Autodesk Inventor part; units mm, degrees
ref_plane "YZ Plane" through (0, 0, 0) normal (1, 0, 0) x (0, 1, 0)
ref_plane "XZ Plane" through (0, 0, 0) normal (0, 1, 0) x (-1, 0, 0)
ref_plane "XY Plane" through (0, 0, 0) normal (0, 0, 1) x (1, 0, 0)
sketch "Boceto1" plane through (0, 0, 0) normal (0, 1, 0) x (-1, 0, 0)
  circle A0 centre (0, 0) radius 5
  circle A1 centre (0, 0) radius 1.5
  dimension "d0" = 10
  dimension "d1" = 3
extrude "Extrusión1" add sketch "Boceto1" along normal blind 10
sketch "Boceto2" plane through (0, 10, 0) normal (0, 1, 0) x (1, 0, 0)
  circle A0 centre (0, 0) radius 11
  circle A1 centre (0, 0) radius 5
  circle A2 centre (0, 0) radius 1.5
  dimension "d4" = 22
extrude "Extrusión2" add sketch "Boceto2" along normal blind 2.2 contours A0 | A1
sketch "Boceto3" plane through (0, 12.2, 0) normal (0, 1, 0) x (1, 0, 0)
  circle A0 centre (0, 0) radius 9.475
  circle A1 centre (0, 0) radius 6.6
  line L0 (0, -6.6) -> (0, -9.475)
  circle A2 centre (0, -8.0375) radius 1.4375
  circle A3 centre (8.0375, 0) radius 1.4375
  circle A4 centre (0, 8.0375) radius 1.4375
  circle A5 centre (-8.0375, 0) radius 1.4375
  dimension "d7" = 18.95
  dimension "d8" = 13.2
  dimension "d11" = 360
hole "Agujero1" at (0, 12.2, 8.0375) at (-8.0375, 12.2, 0) at (0, 12.2, -8.0375) at (8.0375, 12.2, 0) direction (0, -1, 0) diameter 2.85 end through all
properties part number "Acople motor" material "Hierro, dúctil"
The listing builds one solid part. Answer for the finished solid, in the listing's coordinates (mm). A direction names the side the tool comes from. Coordinates: 2 decimals unless noted, no trailing zeros. Loops run counter-clockwise (first coordinate to the right, second up) from the corner with the lowest first, then second, coordinate; pieces in that order, holes last. Notation, with made-up numbers: M 4,-10 L 24,-10 A13 ccw 24,15 Z; hole C -7.5,32 d10. An arc over 180 degrees is marked long. Answer as CSV lines item,"result". Start each with the question number.
(1) For faces 1 (the flat face through (2, 10, 5)), 2 (the flat face through (0, 12.2, 2)), determine the directions among +Z, -Z, +X, -X, +Y, -Y from which every point of the face is accessible in a straight line to the end or side of a thin tool.
(2) Given pin 1 (4 mm diameter, centred on x = -3.5, y = 1.5, fed in from +Z); pin 2 (2 mm diameter, centred on y = 2.5, z = 1.5, fed in from -X); pin 3 (1.5 mm diameter, centred on x = -6.5, z = -8, fed in from -Y); pin 4 (3.5 mm diameter, centred on x = 0, z = 8.04, fed in from +Y), each flat-ended and moving along its own axis, determine where each tip first touches the part or whether it passes through.
(3) Find the intervals of material crossed by L1, parallel to Z at x = 0, y = 10.95; L2, parallel to Z at x = 0, y = 4.25; L3, parallel to Y at x = 6, z = -1, in increasing order. Write a range as [from, to].
(4) The part is cut by section C-C (y = 5). Give the vertices of the cut face in (x, z), and give its area (3 significant figures).
(5) The part is cut by section B-B (z = -4). Give the vertices of the cut face in (x, y).
(6) The mould has two halves that part along Z. Classify faces 3 (the cylindrical face through (9.43, 11.08, -0.31)), 4 (the cylindrical face through (1.08, 4.93, 4.88)), 5 (the flat face through (1.2, 0, 1.2)): pulls with the +Z half, pulls with the -Z half, needs draft (parallel to the pull), parting line crosses it, or undercut.
(7) The part is cut by section D-D (x = -4). Give the vertices of the cut face in (y, z), and give its area (3 significant figures).
Determined:
1,face 1,"-Y"
1,face 2,"+Z, -Z, +X, -X, +Y"
2,pin 1,"z = 4.77"
2,pin 2,"x = -4.97"
2,pin 3,"y = 10"
2,pin 4,"y = 12.2"
3,L1,"[-11, -9.46], [-6.61, -1.5], [1.5, 6.61], [9.46, 11]"
3,L2,"[-5, -1.5], [1.5, 5]"
3,L3,"[10, 12.2]"
4,outline,"C 0,0 d10; hole C 0,0 d3"
4,area,"71.5 mm2"
5,outline,"M -10.25,10 L -3,10 L -3,0 L 3,0 L 3,10 L 10.25,10 L 10.25,12.2 L -10.25,12.2 Z"
6,face 3,"undercut"
6,face 4,"parting line crosses it"
6,face 5,"needs draft"
7,outline,"M 0,-3 L 10,-3 L 10,-10.25 L 12.2,-10.25 L 12.2,10.25 L 10,10.25 L 10,3 L 0,3 Z"
7,area,"105 mm2"
